Here's how the part is built. I have some questions about the finished solid (model axes, mm). A direction names the side the tool comes from. Round coordinates to 2 decimals unless told otherwise and drop trailing zeros. Order: outer loops, then holes, each group sorted by start corner. A loop starts at its lowest first (then second) coordinate and runs counter-clockwise, first axis right, second up. Notation, with made-up numbers: (-15, 23) -> (-4, 23) arc R7 ccw to (-4, 28) -> close; hole circle Ø9 at (-37.5, 73). An arc over 180 degrees is marked (long way). Use a Markdown table: item, result. Add a question column.
(1) On a 3-axis mill with a long thin cutter (end or side, diameter ignored), from which of +Z, -Z, +X, -X, +Y, -Y can I reach the whole of each face in a straight line? I mean faces 5 (the face through (4, 2, 0.5)), 6 (the face through (1.5, 2, -2)), 7 (the face through (1, 0, 0)). Say none if no direction works.
(2) I want a section at D-D, the plane z = -0.5. Please give me the cut outline in (x, y).
(3) If I drill on probe 1 along Z at (x, y) = (4.5, 1.1); probe 2 along X at (y, z) = (1.1, 3); probe 3 along Y at (x, z) = (5.75, -1), over which ranges is the centre line in solid material (lowest first)?
(4) I want a section at C-C, the plane y = 0.95. Please give me the cut outline in (x, z), then the cut area to 3 significant figures.
(5) Thinking about a two-plate mould opening in X: for faces 1 (the face through (-7.5, 0, 0)), 2 (the face through (-6, -2.5, 0)), 3 (the face through (-4.5, -1, 0)), 4 (the face through (3.7, 0.7, 3.6)), which applies, pulls with the +X half, pulls with the -X half, needs draft (parallel to the pull), parting line crosses it, or undercut?
(6) I want a section at B-B, the plane x = 4.5. Please give me the cut outline in (y, z), then the cut area to 3 significant figures.
(7) I'm going to push flat-ended pins straight in: P1, Ø0.8, axis at y = -1, z = -1, coming from the +X side; P2, Ø0.8, axis at x = 3, y = 2, coming from the +Z side; P3, Ø1, axis at x = -3, z = 1.5, coming from the +Y side. Where does each tip first touch, or does it pass through?
(8) I want a section at A-A, the plane z = 3. Please give me the cut outline in (x, y), then the cut area to 3 significant figures.
from build123d import *

# Parameters (mm, degrees)
SKETCH_1_R      = 1
SKETCH_1_W      = 5
SKETCH_1_H      = 5
SKETCH_1_W_2    = 3
SKETCH_1_H_2    = 11
EXTRUDE_1_DEPTH = 1.5
SKETCH_1_3_W    = 3
SKETCH_1_3_H    = 11
EXTRUDE_2_DEPTH = 2.5
EXTRUDE_START   = 1.5
SKETCH_1_4_W    = 5
SKETCH_1_4_H    = 5
EXTRUDE_3_DEPTH = 1.5


with BuildPart() as part:
    # Эскиз1 → Бобышка-Вытянуть1 (new body)
    with BuildSketch(Plane(origin=(0, 0, 0), x_dir=(1, 0, 0), z_dir=(0, 1, 0))):
        Polygon((7.5, -3), (7.5, 5.5), (-4.5, 5.5), (-4.5, -5.5), (4.5, -5.5), (7.5, -5.5), align=None)
        with Locations((4.5, -3)):
            Circle(SKETCH_1_R, mode=Mode.SUBTRACT)
        with Locations((4, 2)):
            Rectangle(SKETCH_1_W, SKETCH_1_H, mode=Mode.SUBTRACT)
        with Locations((-6, 0)):
            Rectangle(SKETCH_1_W_2, SKETCH_1_H_2)
        with Locations((4, 2)):
            Rectangle(SKETCH_1_W, SKETCH_1_H)
    extrude(amount=EXTRUDE_1_DEPTH)

    # Эскиз1<3> → Бобышка-Вытянуть2 (add)
    with BuildSketch(Plane(origin=(0, 0, 0), x_dir=(1, 0, 0), z_dir=(0, 1, 0))):
        with Locations((-6, 0)):
            Rectangle(SKETCH_1_3_W, SKETCH_1_3_H)
    extrude(amount=-EXTRUDE_2_DEPTH)

    # Эскиз1<4> → Бобышка-Вытянуть3 (add)
    with BuildSketch(Plane(origin=(0, 0, 0), x_dir=(1, 0, 0), z_dir=(0, 1, 0)).offset(EXTRUDE_START)):
        with Locations((4, 2)):
            Rectangle(SKETCH_1_4_W, SKETCH_1_4_H)
    extrude(amount=EXTRUDE_3_DEPTH)


solid = part.part
Taken from the geometry:
| question | item | result |
|---|---|---|
| 1 | face 5 | +Z, +X, -X, +Y |
| 1 | face 6 | +Z, -Z, -X, +Y |
| 1 | face 7 | +Z, -Z, +X, -Y |
| 2 | outline | (-7.5, -2.5) -> (-4.5, -2.5) -> (-4.5, 0) -> (7.5, 0) -> (7.5, 1.5) -> (6.5, 1.5) -> (6.5, 3) -> (1.5, 3) -> (1.5, 1.5) -> (-7.5, 1.5) -> close |
| 3 | probe 1 | z = -5.5 to 2, 4 to 5.5 |
| 3 | probe 2 | x = -7.5 to 3.5, 5.5 to 7.5 |
| 3 | probe 3 | y = 0 to 3 |
| 4 | outline | (-7.5, -5.5) -> (7.5, -5.5) -> (7.5, 5.5) -> (-7.5, 5.5) -> close; hole circle Ø2 at (4.5, 3) |
| 4 | area | 162 mm2 |
| 5 | face 1 | pulls with the -X half |
| 5 | face 2 | needs draft |
| 5 | face 3 | pulls with the +X half |
| 5 | face 4 | undercut |
| 6 | outline | (0, -5.5) -> (1.5, -5.5) -> (1.5, -4.5) -> (3, -4.5) -> (3, 0.5) -> (1.5, 0.5) -> (1.5, 2) -> (0, 2) -> close; (0, 4) -> (1.5, 4) -> (1.5, 5.5) -> (0, 5.5) -> close |
| 6 | area | 21.0 mm2 |
| 7 | P1 | stops at x = -4.5 |
| 7 | P2 | stops at z = 0.5 |
| 7 | P3 | stops at y = 1.5 |
| 8 | outline | (-7.5, -2.5) -> (-4.5, -2.5) -> (-4.5, 0) -> (3.5, 0) -> (3.5, 1.5) -> (-7.5, 1.5) -> close; (5.5, 0) -> (7.5, 0) -> (7.5, 1.5) -> (5.5, 1.5) -> close |
| 8 | area | 27.0 mm2 |
